```python
from build123d import *

# Parameters (mm, degrees)
F1_DEPTH   = 80
F2_W       = 20
F2_H       = 3.5
F3_DEPTH   = 4.001
F4_SIZE2   = 11.99999
F4_SIZE    = 5.99999
F5_SIZE2   = 2.5
F5_SIZE    = 15
F5_2_SIZE2 = 2.5
F5_2_SIZE  = 15
F5_3_SIZE2 = 2.5
F5_3_SIZE  = 15
F5_4_SIZE2 = 2.5
F5_4_SIZE  = 15
F5_5_SIZE2 = 2.5
F5_5_SIZE  = 15
F5_6_SIZE2 = 2.5
F5_6_SIZE  = 15
F5_7_SIZE2 = 2.5
F5_7_SIZE  = 15
F5_8_SIZE2 = 2.5
F5_8_SIZE  = 15
F6_SIZE2   = 2.5
F6_SIZE    = 15
F6_2_SIZE2 = 2.5
F6_2_SIZE  = 15
F6_3_SIZE2 = 2.5
F6_3_SIZE  = 15
F6_4_SIZE2 = 2.5
F6_4_SIZE  = 15
F6_5_SIZE2 = 2.5
F6_5_SIZE  = 15
F6_6_SIZE2 = 2.5
F6_6_SIZE  = 15
F6_7_SIZE2 = 2.5
F6_7_SIZE  = 15
F6_8_SIZE2 = 2.5
F6_8_SIZE  = 15
F7_W       = 30
F7_H       = 80
F8_DEPTH   = 25
F9_W       = 12
F9_H       = 12
F10_DEPTH  = 10.001


# Not quite as in the source:
# - a fillet or chamfer is up to 0.001 mm smaller than in the source, because OpenCascade refuses the exact size


with BuildPart() as f1:
    # F0 (on Front) → F1 (new body)
    with BuildSketch(Plane.XZ):
        Polygon((0, 4), (0, 0), (32, 0), (32, 6), (100, 6), (100, 10), (20, 10), (20, 4), align=None)
    extrude(amount=F1_DEPTH)

    # F2 (on face) → F3 (cut, through all)
    with BuildSketch(Plane.XY.offset(4)):
        with Locations((10, -35.5)):
            Rectangle(F2_W, F2_H)
        with Locations((10, -26.5)):
            Rectangle(F2_W, F2_H)
        with Locations((10, -17.5)):
            Rectangle(F2_W, F2_H)
        with Locations((10, -8.5)):
            Rectangle(F2_W, F2_H)
        with Locations((10, -71.5)):
            Rectangle(F2_W, F2_H)
        with Locations((10, -53.5)):
            Rectangle(F2_W, F2_H)
        with Locations((10, -44.5)):
            Rectangle(F2_W, F2_H)
        with Locations((10, -62.5)):
            Rectangle(F2_W, F2_H)
    extrude(amount=-F3_DEPTH, mode=Mode.SUBTRACT)

    # F4 (size 6 and 12 in the source; OpenCascade refuses exactly that, so slightly less here)
    f4_edges = [f1.edges().sort_by_distance(p)[0] for p in [
        (20, -40, 10),
    ]]
    f4_side = f1.faces().sort_by_distance((20, -40, 6.054054))[0]
    chamfer(f4_edges, length=F4_SIZE, length2=F4_SIZE2, reference=f4_side)

    # F5
    f5_edges = [f1.edges().sort_by_distance(p)[0] for p in [
        (0, -6.75, 2),
    ]]
    f5_side = f1.faces().sort_by_distance((10, -6.75, 2))[0]
    chamfer(f5_edges, length=F5_SIZE, length2=F5_SIZE2, reference=f5_side)

    # F5#2
    f5_2_edges = [f1.edges().sort_by_distance(p)[0] for p in [
        (0, -69.75, 2),
    ]]
    f5_2_side = f1.faces().sort_by_distance((10, -69.75, 2))[0]
    chamfer(f5_2_edges, length=F5_2_SIZE, length2=F5_2_SIZE2, reference=f5_2_side)

    # F5#3
    f5_3_edges = [f1.edges().sort_by_distance(p)[0] for p in [
        (0, -15.75, 2),
    ]]
    f5_3_side = f1.faces().sort_by_distance((10, -15.75, 2))[0]
    chamfer(f5_3_edges, length=F5_3_SIZE, length2=F5_3_SIZE2, reference=f5_3_side)

    # F5#4
    f5_4_edges = [f1.edges().sort_by_distance(p)[0] for p in [
        (0, -60.75, 2),
    ]]
    f5_4_side = f1.faces().sort_by_distance((10, -60.75, 2))[0]
    chamfer(f5_4_edges, length=F5_4_SIZE, length2=F5_4_SIZE2, reference=f5_4_side)

    # F5#5
    f5_5_edges = [f1.edges().sort_by_distance(p)[0] for p in [
        (0, -24.75, 2),
    ]]
    f5_5_side = f1.faces().sort_by_distance((10, -24.75, 2))[0]
    chamfer(f5_5_edges, length=F5_5_SIZE, length2=F5_5_SIZE2, reference=f5_5_side)

    # F5#6
    f5_6_edges = [f1.edges().sort_by_distance(p)[0] for p in [
        (0, -51.75, 2),
    ]]
    f5_6_side = f1.faces().sort_by_distance((10, -51.75, 2))[0]
    chamfer(f5_6_edges, length=F5_6_SIZE, length2=F5_6_SIZE2, reference=f5_6_side)

    # F5#7
    f5_7_edges = [f1.edges().sort_by_distance(p)[0] for p in [
        (0, -33.75, 2),
    ]]
    f5_7_side = f1.faces().sort_by_distance((10, -33.75, 2))[0]
    chamfer(f5_7_edges, length=F5_7_SIZE, length2=F5_7_SIZE2, reference=f5_7_side)

    # F5#8
    f5_8_edges = [f1.edges().sort_by_distance(p)[0] for p in [
        (0, -42.75, 2),
    ]]
    f5_8_side = f1.faces().sort_by_distance((10, -42.75, 2))[0]
    chamfer(f5_8_edges, length=F5_8_SIZE, length2=F5_8_SIZE2, reference=f5_8_side)

    # F6
    f6_edges = [f1.edges().sort_by_distance(p)[0] for p in [
        (0, -37.25, 2),
    ]]
    f6_side = f1.faces().sort_by_distance((10, -37.25, 2))[0]
    chamfer(f6_edges, length=F6_SIZE, length2=F6_SIZE2, reference=f6_side)

    # F6#2
    f6_2_edges = [f1.edges().sort_by_distance(p)[0] for p in [
        (0, -46.25, 2),
    ]]
    f6_2_side = f1.faces().sort_by_distance((10, -46.25, 2))[0]
    chamfer(f6_2_edges, length=F6_2_SIZE, length2=F6_2_SIZE2, reference=f6_2_side)

    # F6#3
    f6_3_edges = [f1.edges().sort_by_distance(p)[0] for p in [
        (0, -28.25, 2),
    ]]
    f6_3_side = f1.faces().sort_by_distance((10, -28.25, 2))[0]
    chamfer(f6_3_edges, length=F6_3_SIZE, length2=F6_3_SIZE2, reference=f6_3_side)

    # F6#4
    f6_4_edges = [f1.edges().sort_by_distance(p)[0] for p in [
        (0, -55.25, 2),
    ]]
    f6_4_side = f1.faces().sort_by_distance((10, -55.25, 2))[0]
    chamfer(f6_4_edges, length=F6_4_SIZE, length2=F6_4_SIZE2, reference=f6_4_side)

    # F6#5
    f6_5_edges = [f1.edges().sort_by_distance(p)[0] for p in [
        (0, -19.25, 2),
    ]]
    f6_5_side = f1.faces().sort_by_distance((10, -19.25, 2))[0]
    chamfer(f6_5_edges, length=F6_5_SIZE, length2=F6_5_SIZE2, reference=f6_5_side)

    # F6#6
    f6_6_edges = [f1.edges().sort_by_distance(p)[0] for p in [
        (0, -64.25, 2),
    ]]
    f6_6_side = f1.faces().sort_by_distance((10, -64.25, 2))[0]
    chamfer(f6_6_edges, length=F6_6_SIZE, length2=F6_6_SIZE2, reference=f6_6_side)

    # F6#7
    f6_7_edges = [f1.edges().sort_by_distance(p)[0] for p in [
        (0, -10.25, 2),
    ]]
    f6_7_side = f1.faces().sort_by_distance((10, -10.25, 2))[0]
    chamfer(f6_7_edges, length=F6_7_SIZE, length2=F6_7_SIZE2, reference=f6_7_side)

    # F6#8
    f6_8_edges = [f1.edges().sort_by_distance(p)[0] for p in [
        (0, -73.25, 2),
    ]]
    f6_8_side = f1.faces().sort_by_distance((10, -73.25, 2))[0]
    chamfer(f6_8_edges, length=F6_8_SIZE, length2=F6_8_SIZE2, reference=f6_8_side)

    # F7 (on face) → F8 (cut)
    with BuildSketch(Plane.XY.offset(10)):
        with Locations((85, -40)):
            Rectangle(F7_W, F7_H)
    extrude(amount=-F8_DEPTH, mode=Mode.SUBTRACT)

    # F9 (on face) → F10 (cut, through all)
    with BuildSketch(Plane.XY.offset(10)):
        with Locations((41.5, -10)):
            Rectangle(F9_W, F9_H)
        with Locations((41.5, -30)):
            Rectangle(F9_W, F9_H)
        with Locations((41.5, -50)):
            Rectangle(F9_W, F9_H)
        with Locations((41.5, -70)):
            Rectangle(F9_W, F9_H)
        with Locations((60.5, -30)):
            Rectangle(F9_W, F9_H)
        with Locations((60.5, -70)):
            Rectangle(F9_W, F9_H)
        with Locations((60.5, -10)):
            Rectangle(F9_W, F9_H)
        with Locations((60.5, -50)):
            Rectangle(F9_W, F9_H)
    extrude(amount=-F10_DEPTH, mode=Mode.SUBTRACT)


solid = f1.part
```
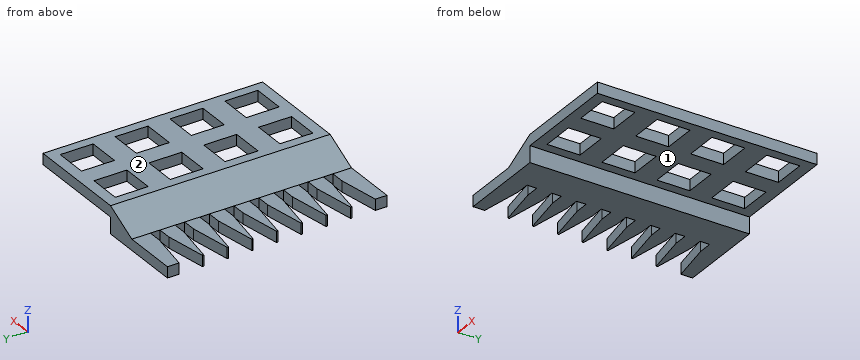
Source: CAD feature listing. Evaluate the final solid. Frame: model axes, mm. Face numbers are marked on the shaded views. A direction names the side the tool comes from. Give positions to 0.01 mm unless a question says otherwise; leave off trailing zeros. Order: outer loops, then holes, each group sorted by start corner. A loop starts at its lowest first (then second) coordinate and runs counter-clockwise, first axis right, second up.
(1) Section query D-D (x = 10). State how many separate pieces and enclosed holes the cut face has, plus the area to 3 significant figures.
(2) Access query for the marked faces 1 and 2. Directions: +Z, -Z, +X, -X, +Y, -Y. A direction counts if a zero-diameter tool reaches every point of the face in a straight line with its end or side. Return the directions, or none.
(3) Section query C-C (y = -62.5). Return the cut outline in (x, z), plus the area to 3 significant figures.
(4) Material intervals for line 1 along Y through (x, z) = (60.5, 6.25); line 2 along X through (y, z) = (-46.5, 8.25); line 3 along X through (y, z) = (-31, 8.5), sorted ascending.
(5) Section query B-B (y = -27). Return the cut outline in (x, z).
(6) Section query A-A (x = 44). Return the cut outline in (y, z).
(7) Contact query for flat-ended pins moving along their axis: P1, Ø5, axis at x = 46.5, y = -69, coming from the -Z side; P2, Ø6, axis at x = 7.5, y = -31, coming from the +Z side; P3, Ø10, axis at x = 18.5, y = -25.5, coming from the +Z side. Output: stop coordinate, or through.
Outcome:
1. separate pieces: 9
1. enclosed holes: 0
1. area: 155 mm2
2. face 1: -Z, +X, +Y, -Y
2. face 2: +Z, +X, -X, +Y, -Y
3. outline: (20, 0) - (32, 0) - (32, 6) - (70, 6) - (70, 10) - (32, 10) - (20, 4) - close
3. area: 236 mm2
4. line 1: y = -80 to -76, -64 to -56, -44 to -36, -24 to -16, -4 to 0
4. line 2: x = 28.5 to 35.5, 47.5 to 54.5, 66.5 to 70
4. line 3: x = 29 to 35.5, 47.5 to 54.5, 66.5 to 70
5. outline: (20, 0) - (32, 0) - (32, 6) - (35.5, 6) - (35.5, 10) - (32, 10) - (20, 4) - close; (47.5, 6) - (54.5, 6) - (54.5, 10) - (47.5, 10) - close; (66.5, 6) - (70, 6) - (70, 10) - (66.5, 10) - close
6. outline: (-80, 6) - (-76, 6) - (-76, 10) - (-80, 10) - close; (-64, 6) - (-56, 6) - (-56, 10) - (-64, 10) - close; (-44, 6) - (-36, 6) - (-36, 10) - (-44, 10) - close; (-24, 6) - (-16, 6) - (-16, 10) - (-24, 10) - close; (-4, 6) - (0, 6) - (0, 10) - (-4, 10) - close
7. P1: stops at z = 6
7. P2: stops at z = 4
7. P3: stops at z = 5.75
